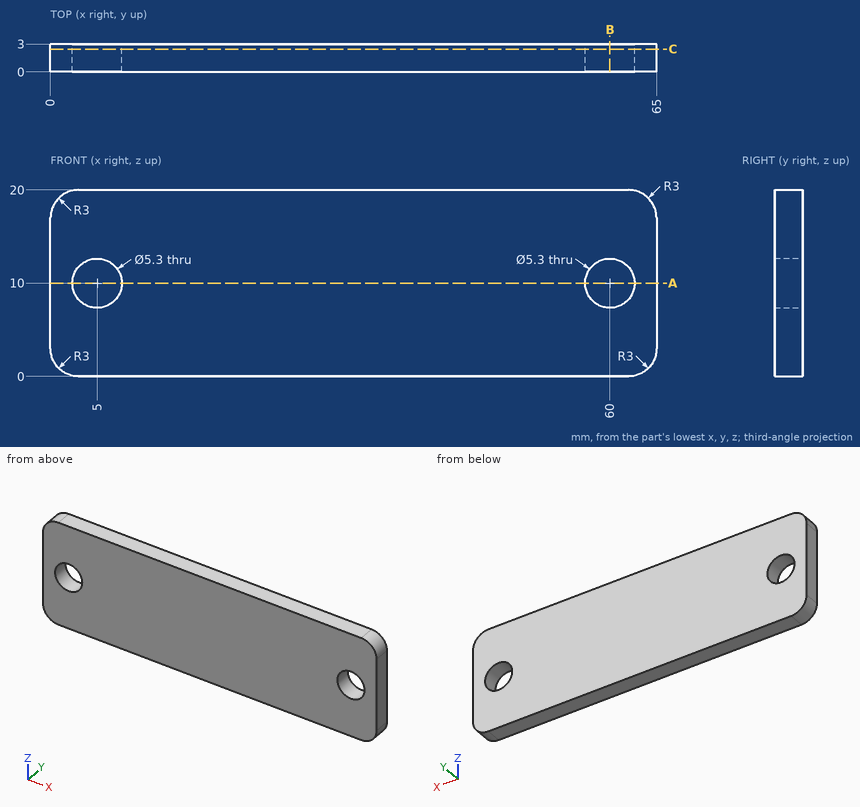
Design review of the part shown in the three views and the two pictorial views. Dimensions are in mm from the part's minimum x, y and z. Round coordinates to 2 decimals unless told otherwise and drop trailing zeros. Write each loop counter-clockwise with the first axis right and the second up, starting at its lowest first coordinate (ties: lowest second). Pieces come first, ordered by that corner, then holes.
1) Take a section at B-B on x = 60. Give the boundary of the cut face in (y, z).
Answer below:
outline: (0, 0) - (3, 0) - (3, 7.35) - (0, 7.35) - close; (0, 12.65) - (3, 12.65) - (3, 20) - (0, 20) - close
2) Take a section at C-C on y = 2.45. Give the boundary of the cut face in (x, z), then the cut area to 3 significant figures.
Answer below:
outline: (0, 3) arc R3 ccw to (3, 0) - (62, 0) arc R3 ccw to (65, 3) - (65, 17) arc R3 ccw to (62, 20) - (3, 20) arc R3 ccw to (0, 17) - close; hole circle Ø5.3 at (5, 10); hole circle Ø5.3 at (60, 10)
area: 1,250 mm2
3) For line 1 along X through (y, z) = (2.3, 10); line 2 along Z through (x, y) = (60, 1.25); line 3 along X through (y, z) = (0.6, 11), list the stretches that pass through material, from the lowest coordinate up.
Answer below:
line 1: x = 0 to 2.35, 7.65 to 57.35, 62.65 to 65
line 2: z = 0 to 7.35, 12.65 to 20
line 3: x = 0 to 2.55, 7.45 to 57.55, 62.45 to 65
4) Take a section at A-A on z = 10. Give the boundary of the cut face in (x, y), then the cut area to 3 significant figures.
Answer below:
outline: (0, 0) - (2.35, 0) - (2.35, 3) - (0, 3) - close; (7.65, 0) - (57.35, 0) - (57.35, 3) - (7.65, 3) - close; (62.65, 0) - (65, 0) - (65, 3) - (62.65, 3) - close
area: 163 mm2
